from build123d import *

# Parameters (mm, degrees)
SKETCH1_W              = 44.45
SKETCH1_H              = 25.4
BOSS_EXTRUDE1_DEPTH    = 57.15
CUT_EXTRUDE1_REACH     = 64.621
SKETCH2_R              = 4.7625
F_12_CLEARANCE_HOLE1_D = 5.7912


with BuildPart() as part:
    # Sketch1 → Boss-Extrude1 (new body)
    with BuildSketch(Plane(origin=(0, 0, 0), x_dir=(1, 0, 0), z_dir=(0, 1, 0))):
        Rectangle(SKETCH1_W, SKETCH1_H)
    extrude(amount=BOSS_EXTRUDE1_DEPTH)

    # Sketch2 → Cut-Extrude1 (cut, up to next)
    with BuildSketch(Plane(origin=(0, 57.15, 0), x_dir=(1, 0, 0), z_dir=(0, 1, 0)), mode=Mode.PRIVATE) as cut_extrude1_sk1:
        with Locations(Location((0, 0, 0), (0, 0, 270))):
            Circle(SKETCH2_R)
    cut_extrude1_tool1 = extrude(cut_extrude1_sk1.sketch, amount=-CUT_EXTRUDE1_REACH, mode=Mode.PRIVATE) & part.part
    add(cut_extrude1_tool1.solids().sort_by_distance((0, 57.15, 0))[0], mode=Mode.SUBTRACT)

    # #12 Clearance Hole1 (through all)
    with Locations(Plane.XY.offset(12.7)):
        with Locations((-18.25625, 51.5874), (18.25625, 29.3624), (-18.25625, 29.3624), (18.25625, 51.5874)):
            Hole(F_12_CLEARANCE_HOLE1_D / 2)


solid = part.part
Can you work these out from the model? Positions are in its coordinate system, mm. Coordinates: 2 decimals unless noted, no trailing zeros. Loops run counter-clockwise (first coordinate to the right, second up) from the corner with the lowest first, then second, coordinate; pieces in that order, holes last. Notation, with made-up numbers: (11, 9.25) - (42, 9.25) arc R27 ccw to (42, 40.25) - close; hole circle Ø6 at (2, 39). An arc over 180 degrees is marked (long way). Put each result on its own line as item: value. Start each with the question number.
Item 1: Suppose I cut it at D-D (z = -7.5). Please give me the cut outline in (x, y) (3 decimals), and give its area (3 significant figures).
Item 2: Suppose I cut it at C-C (z = 0). State how many separate pieces and enclosed holes the cut face has, and give its area (3 significant figures).
Item 3: Suppose I cut it at A-A (x = 0). Please give me the cut outline in (y, z).
Item 4: If I drill on line 1 along Y through (x, z) = (18, -9.25); line 2 along Y through (x, z) = (16, 6.5); line 3 along X through (y, z) = (31, -8.75) (3 decimals), over which ranges is the centre line in solid material (lowest first)?
Item 5: Suppose I cut it at B-B (y = 15.5). Please give me the cut outline in (x, z) (1 decimal).
Item 6: If we mould it in two halves opening along Y, with no side actions, what happens to faces 1 (the face through (20.554, 49.825, -0.178)), 2 (the face through (-5, 0, 0)), 3 (the face through (-22.225, 28, 0))? For each: +Y half, -Y half, draft (parallel to the pull), parting line (faces both ways), or undercut.
Item 7: For pin 1 (8 mm diameter, centred on x = -11.5, z = 5.5, fed in from -Y); pin 2 (5 mm diameter, centred on x = 18.26, y = 51.59, fed in from +Z), each with a flat end and sliding along its axis, tell me the tip position at first contact or that it passes through.
Here are the results:
1. outline: (-22.225, 0) - (22.225, 0) - (22.225, 57.15) - (-22.225, 57.15) - close; hole circle Ø5.791 at (-18.256, 29.362); hole circle Ø5.791 at (-18.256, 51.587); hole circle Ø5.791 at (18.256, 29.362); hole circle Ø5.791 at (18.256, 51.587)
1. area: 2,430 mm²
2. separate pieces: 2
2. enclosed holes: 4
2. area: 1,890 mm²
3. outline: (0, -12.7) - (57.15, -12.7) - (57.15, -4.76) - (0, -4.76) - close; (0, 4.76) - (57.15, 4.76) - (57.15, 12.7) - (0, 12.7) - close
4. line 1: 0 to 26.48, 32.25 to 48.7, 54.47 to 57.15
4. line 2: 0 to 27.55, 31.18 to 49.77, 53.4 to 57.15
4. line 3: -22.225 to -20.644, -15.868 to 15.868, 20.644 to 22.225
5. outline: (-22.2, -12.7) - (22.2, -12.7) - (22.2, 12.7) - (-22.2, 12.7) - close; hole circle Ø9.5 at (0, 0)
6. face 1: undercut
6. face 2: -Y half
6. face 3: draft
7. pin 1: y = 0
7. pin 2: through
